```python
from build123d import *

# Parameters (mm, degrees)
SKETCH1_W           = 54.1782
SKETCH1_H           = 76.2
BOSS_EXTRUDE1_DEPTH = 5.461
SKETCH2_W           = 12.7
SKETCH2_H           = 5.461
SKETCH2_W_2         = 38.1
SKETCH2_H_2         = 12.7
BOSS_EXTRUDE2_DEPTH = 5.461
SKETCH3_W           = 5.461
SKETCH3_H           = 25.4
CUT_EXTRUDE1_DEPTH  = 6.461


with BuildPart() as part:
    # Sketch1 → Boss-Extrude1 (new body)
    with BuildSketch(Plane(origin=(0, 0, 0), x_dir=(1, 0, 0), z_dir=(0, 1, 0))):
        Rectangle(SKETCH1_W, SKETCH1_H)
    extrude(amount=BOSS_EXTRUDE1_DEPTH)

    # Sketch2 → Boss-Extrude2 (add)
    with BuildSketch(Plane(origin=(0, 5.461, 0), x_dir=(1, 0, 0), z_dir=(0, 1, 0))):
        with Locations((-15.875, -40.8305)):
            Rectangle(SKETCH2_W, SKETCH2_H)
        with Locations((15.875, -40.8305)):
            Rectangle(SKETCH2_W, SKETCH2_H)
        with Locations((0, 44.45)):
            Rectangle(SKETCH2_W_2, SKETCH2_H_2)
    extrude(amount=-BOSS_EXTRUDE2_DEPTH)

    # Sketch3 → Cut-Extrude1 (cut, through all)
    with BuildSketch(Plane(origin=(0, 5.461, 0), x_dir=(1, 0, 0), z_dir=(0, 1, 0))):
        with Locations((-24.3586, 0)):
            Rectangle(SKETCH3_W, SKETCH3_H)
        with Locations((24.3586, 0)):
            Rectangle(SKETCH3_W, SKETCH3_H)
    extrude(amount=-CUT_EXTRUDE1_DEPTH, mode=Mode.SUBTRACT)


solid = part.part
```
Can you work these out from the model? Positions are in its coordinate system, mm. A direction names the side the tool comes from. Coordinates: 2 decimals unless noted, no trailing zeros. Order: outer loops, then holes, each group sorted by start corner. A loop starts at its lowest first (then second) coordinate and runs counter-clockwise, first axis right, second up.
1. If we section it at A-A (y = 2): Please give me the cut outline in (x, z) (3 decimals), then the cut area to 3 significant figures.
2. For faces 1 (the face through (-9.525, 3, 41)), 2 (the face through (21.628, 3, 0)), 3 (the face through (-25, 3, 38.1)), 4 (the face through (-24, 3, -12.7)), 5 (the face through (23, 3, -38.1)), which set-ups out of +Z, -Z, +X, -X, +Y, -Y let a thin tool reach every point of the face, with its end or its side?
3. If we section it at B-B (z = 6): Please give me the cut outline in (x, y).
4. I'm going to push flat-ended pins straight in: pin 1 (1.6 mm diameter, centred on x = 25.5, y = 3, fed in from +Z); pin 2 (2.5 mm diameter, centred on x = 22.5, y = 2, fed in from -Z); pin 3 (1.6 mm diameter, centred on y = 3, z = -1.5, fed in from -X). Where does each tip first touch, or does it pass through?
5. If we section it at C-C (x = -4): Please give me the cut outline in (y, z), then the cut area to 3 significant figures.
6. Thinking about a two-plate mould opening in Z: for faces 6 (the face through (27.089, 3, 26)), 7 (the face through (0, 3, 38.1)), 8 (the face through (-24, 3, 12.7)), which applies, +Z half, -Z half, draft (parallel to the pull), parting line (faces both ways), or undercut?
7. I need wall thicknesses on line 1 (Z direction, x = 24, y = 1.8); line 2 (X direction, y = 1.3, z = -5.5); line 3 (Z direction, x = -8, y = 4.7). Which ranges of each line are inside material? Lowest first, please.
Entries:
1. outline: (-27.089, -38.1) - (-19.05, -38.1) - (-19.05, -50.8) - (19.05, -50.8) - (19.05, -38.1) - (27.089, -38.1) - (27.089, -12.7) - (21.628, -12.7) - (21.628, 12.7) - (27.089, 12.7) - (27.089, 38.1) - (22.225, 38.1) - (22.225, 43.561) - (9.525, 43.561) - (9.525, 38.1) - (-9.525, 38.1) - (-9.525, 43.561) - (-22.225, 43.561) - (-22.225, 38.1) - (-27.089, 38.1) - (-27.089, 12.7) - (-21.628, 12.7) - (-21.628, -12.7) - (-27.089, -12.7) - close
1. area: 4,470 mm2
2. face 1: +Z, +Y, -Y
2. face 2: +X, +Y, -Y
2. face 3: +Z, -X, +Y, -Y
2. face 4: -X, +Y, -Y
2. face 5: -Z, +X, +Y, -Y
3. outline: (-21.63, 0) - (21.63, 0) - (21.63, 5.46) - (-21.63, 5.46) - close
4. pin 1: stops at z = 38.1
4. pin 2: stops at z = -38.1
4. pin 3: stops at x = -21.63
5. outline: (0, -50.8) - (5.46, -50.8) - (5.46, 38.1) - (0, 38.1) - close
5. area: 485 mm2
6. face 6: draft
6. face 7: +Z half
6. face 8: undercut
7. line 1: z = -38.1 to -12.7, 12.7 to 38.1
7. line 2: x = -21.63 to 21.63
7. line 3: z = -50.8 to 38.1
